Design review of the part built by this model. Coordinates are the model's own, in mm. A direction names the side the tool comes from. Coordinates: 2 decimals unless noted, no trailing zeros. Write each loop counter-clockwise with the first axis right and the second up, starting at its lowest first coordinate (ties: lowest second). Pieces come first, ordered by that corner, then holes.
Q1. The part is to be moulded in two halves that separate along Y. For faces 4 (the flat face through (48, -20.638, 2)), 5 (the flat face through (46.038, 2, 2)), 6 (the flat face through (48, -7.938, 2)), 7 (the flat face through (44.45, -23, 2)), say which applies: released by +Y, released by -Y, zero draft, split by the parting line, or undercut.
Q2. Take a section at C-C, the plane y = 11. Write out the cut boundary in (x, z).
Q3. For pin 1 Ø2.5 at (x, z) = (49, 2) entering from -Y; pin 2 Ø1.4 at (y, z) = (-0.5, 3) entering from -X, all flat-tipped, find the tip position at first contact; note any pin that passes through.
Q4. For L1, parallel to X at y = -21, z = 4.4; L2, parallel to Y at x = -44.5, z = 1; L3, parallel to X at y = 8, z = 1.7, list the stretches that pass through material, from the lowest coordinate up.
Q5. Take a section at A-A, the plane z = 1.6. Write out the cut boundary in (x, y).
Q6. For faces 1 (the flat face through (48, 12.7, 2)), 2 (the flat face through (25, -20.638, 2)), 3 (the flat face through (-46.038, 2, 2)), list the 3-axis set-ups (+Z, -Z, +X, -X, +Y, -Y) from which the entire face can be reached by the end or side of a thin tool; tool diameter is ignored.
Q7. Take a section at B-B, the plane x = 22.5. Write out the cut boundary in (y, z).
from build123d import *

# Parameters (mm, degrees)
F0_W     = 101.6
F0_H     = 50.8
F1_DEPTH = 4.7625
F2_W     = 6.35
F2_H     = 4.7625
F2_W_2   = 12.7
F3_DEPTH = 25.4
F4_W     = 4.7625
F4_H     = 20.6375
F5_DEPTH = 25.4


with BuildPart() as f1:
    # F0 (on Top) → F1 (new body)
    with BuildSketch(Plane.XY):
        Rectangle(F0_W, F0_H)
    extrude(amount=F1_DEPTH)

    # F2 (on face) → F3 (cut)
    with BuildSketch(Plane.XY.offset(4.7625)):
        with Locations((-47.625, -23.01875)):
            Rectangle(F2_W, F2_H)
        with Locations((-25.4, -23.01875)):
            Rectangle(F2_W_2, F2_H)
        with Locations((0, -23.01875)):
            Rectangle(F2_W_2, F2_H)
        with Locations((25.4, -23.01875)):
            Rectangle(F2_W_2, F2_H)
        with Locations((47.625, -23.01875)):
            Rectangle(F2_W, F2_H)
    extrude(amount=-F3_DEPTH, mode=Mode.SUBTRACT)

    # F4 (on face) → F5 (cut)
    with BuildSketch(Plane.XY.offset(4.7625)):
        with Locations((-48.41875, 2.38125)):
            Rectangle(F4_W, F4_H)
        with Locations((48.41875, 2.38125)):
            Rectangle(F4_W, F4_H)
    extrude(amount=-F5_DEPTH, mode=Mode.SUBTRACT)


solid = f1.part
Responses:
1. face 4: released by -Y
1. face 5: undercut
1. face 6: undercut
1. face 7: zero draft
2. outline: (-46.04, 0) - (46.04, 0) - (46.04, 4.76) - (-46.04, 4.76) - close
3. pin 1: stops at y = -20.64
3. pin 2: stops at x = -46.04
4. L1: x = -44.45 to -31.75, -19.05 to -6.35, 6.35 to 19.05, 31.75 to 44.45
4. L2: y = -20.64 to 25.4
4. L3: x = -46.04 to 46.04
5. outline: (-50.8, -20.64) - (-44.45, -20.64) - (-44.45, -25.4) - (-31.75, -25.4) - (-31.75, -20.64) - (-19.05, -20.64) - (-19.05, -25.4) - (-6.35, -25.4) - (-6.35, -20.64) - (6.35, -20.64) - (6.35, -25.4) - (19.05, -25.4) - (19.05, -20.64) - (31.75, -20.64) - (31.75, -25.4) - (44.45, -25.4) - (44.45, -20.64) - (50.8, -20.64) - (50.8, -7.94) - (46.04, -7.94) - (46.04, 12.7) - (50.8, 12.7) - (50.8, 25.4) - (-50.8, 25.4) - (-50.8, 12.7) - (-46.04, 12.7) - (-46.04, -7.94) - (-50.8, -7.94) - close
6. face 1: +Z, -Z, +X
6. face 2: +Z, -Z, -Y
6. face 3: +Z, -Z, -X
7. outline: (-20.64, 0) - (25.4, 0) - (25.4, 4.76) - (-20.64, 4.76) - close
